```python
from build123d import *

# Parameters (mm, degrees)
SKETCH_1_R          = 10
EXTRUDE_1_DEPTH     = 3
SKETCH_2_R          = 1.5
CUT_EXTRUDE_1_DEPTH = 15.45683229480096
EXTRUDE_START       = 12.9
SKETCH_3_R          = 4.5
SKETCH_3_R_2        = 1.5000000000000002
EXTRUDE_2_DEPTH     = 12.9
EXTRUDE_START_2     = -15.9
SKETCH_4_R          = 1.5000000000000002
EXTRUDE_4_DEPTH     = 15.9
EXTRUDE_5_DEPTH     = 5
SKETCH_6_R          = 1.4999999999999751
CUT_EXTRUDE_2_DEPTH = 69.71105565006431
EXTRUDE_START_3     = 5
EXTRUDE_8_DEPTH     = 5
FILLET_1_R          = 10
FILLET_2_R          = 2
SKETCH_8_R          = 3.75
CUT_EXTRUDE_3_DEPTH = 3


with BuildPart() as part:
    # 草图1 → 凸台-拉伸1 (new body)
    with BuildSketch(Plane.XY):
        Circle(SKETCH_1_R)
    extrude(amount=EXTRUDE_1_DEPTH)

    # 草图2 → 切除-拉伸1 (cut, through all)
    with BuildSketch(Plane.XY.offset(3)):
        with BuildLine():
            ThreePointArc((-3.4499999999999966, 4.9499999999999975), (-6.010660171779826, 6.010660171779813), (-4.949999999999979, 3.4499999999999966))
            Line((-4.9499999999999975, 3.4499999999999966), (-4.9499999999999975, 4.949999999999997))
            Line((-4.9499999999999975, 4.9499999999999975), (-3.4499999999999957, 4.9499999999999975))
        make_face()
        with BuildLine():
            Line((-4.9499999999999975, 4.949999999999997), (-4.9499999999999975, 3.4499999999999966))
            ThreePointArc((-4.949999999999979, 3.4499999999999966), (-3.8893398282201694, 3.889339828220182), (-3.4499999999999966, 4.9499999999999975))
            Line((-3.4499999999999957, 4.9499999999999975), (-4.9499999999999975, 4.9499999999999975))
        make_face()
        with BuildLine():
            ThreePointArc((3.450000000000002, 4.95), (3.889339828220187, 3.889339828220172), (4.9500000000000215, 3.4499999999999993))
            Line((4.950000000000003, 3.4499999999999984), (4.950000000000003, 4.95))
            Line((4.950000000000003, 4.95), (3.450000000000002, 4.95))
        make_face()
        with BuildLine():
            Line((4.950000000000003, 4.95), (4.950000000000003, 3.4499999999999984))
            ThreePointArc((4.9500000000000215, 3.4499999999999993), (6.010660171779831, 3.8893398282201845), (6.450000000000004, 4.95))
            ThreePointArc((6.450000000000004, 4.95), (4.950000000000003, 6.450000000000001), (3.450000000000002, 4.95))
            Line((3.450000000000002, 4.95), (4.950000000000003, 4.95))
        make_face()
        with BuildLine():
            ThreePointArc((-4.949999999999978, -3.450000000000001), (-6.0106601717798265, -6.010660171779817), (-3.4499999999999966, -4.950000000000002))
            Line((-3.4499999999999957, -4.950000000000002), (-4.9499999999999975, -4.950000000000002))
            Line((-4.9499999999999975, -4.950000000000002), (-4.9499999999999975, -3.450000000000001))
        make_face()
        with BuildLine():
            Line((-4.9499999999999975, -4.950000000000002), (-3.4499999999999957, -4.950000000000002))
            ThreePointArc((-3.4499999999999966, -4.950000000000002), (-3.8893398282201685, -3.889339828220187), (-4.949999999999978, -3.450000000000001))
            Line((-4.9499999999999975, -3.450000000000001), (-4.9499999999999975, -4.950000000000002))
        make_face()
        with BuildLine():
            ThreePointArc((4.950000000000022, -3.4499999999999993), (3.889339828220188, -3.8893398282201717), (3.450000000000002, -4.95))
            Line((3.450000000000002, -4.95), (4.950000000000003, -4.95))
            Line((4.950000000000003, -4.95), (4.950000000000003, -3.4499999999999993))
        make_face()
        with BuildLine():
            Line((4.950000000000003, -4.95), (3.450000000000002, -4.95))
            ThreePointArc((3.450000000000002, -4.95), (4.950000000000003, -6.450000000000001), (6.450000000000004, -4.95))
            ThreePointArc((6.450000000000004, -4.95), (6.010660171779832, -3.8893398282201854), (4.950000000000022, -3.4499999999999993))
            Line((4.950000000000003, -3.4499999999999993), (4.950000000000003, -4.95))
        make_face()
        Circle(SKETCH_2_R)
    extrude(amount=-CUT_EXTRUDE_1_DEPTH, mode=Mode.SUBTRACT)

    # 草图3 → 凸台-拉伸2 (add)
    with BuildSketch(Plane.XY.offset(3).offset(EXTRUDE_START)):
        with Locations(Location((0, 0, 0), (0, 0, 180))):
            Circle(SKETCH_3_R)
        Circle(SKETCH_3_R_2, mode=Mode.SUBTRACT)
    extrude(amount=-EXTRUDE_2_DEPTH)

    # 草图4 → 凸台-拉伸4 (add)
    with BuildSketch(Plane(origin=(0, 0, 0), x_dir=(-1, 0, 0), z_dir=(0, 0, -1)).offset(EXTRUDE_START_2)):
        Circle(SKETCH_4_R)
    extrude(amount=EXTRUDE_4_DEPTH)

    # 草图5 → 凸台-拉伸5 (add)
    with BuildSketch(Plane.XY.offset(15.9)):
        Polygon((64.59529016246847, -5.1146065812479), (63.94313316774814, -10.575805282470675), (-0.5983060285210257, -2.8684953448666564), (0.05385096619931135, 2.5927033563560817), align=None)
    extrude(amount=EXTRUDE_5_DEPTH)

    # 草图6 → 切除-拉伸2 (cut, through all)
    with BuildSketch(Plane.XY.offset(20.900000000000002)):
        with Locations((59.55641321806875, -7.28242024320529)):
            Circle(SKETCH_6_R)
    extrude(amount=-CUT_EXTRUDE_2_DEPTH, mode=Mode.SUBTRACT)

    # 草图7 → 凸台-拉伸8 (add)
    with BuildSketch(Plane.XY.offset(15.9).offset(EXTRUDE_START_3)):
        with BuildLine():
            Line((0.05385096619931135, 2.5927033563560817), (3.9664004294167037, 2.1254805653129325))
            ThreePointArc((3.9664004294167037, 2.1254805653129325), (-4.4378387444626375, 0.7453772723569406), (3.054352769395848, -3.3046829136974565))
            Line((3.054352769395848, -3.3046829136974565), (-0.5983060285210257, -2.8684953448666564))
            Line((-0.5983060285210257, -2.8684953448666564), (0.05385096619931135, 2.5927033563560817))
        make_face()
    extrude(amount=-EXTRUDE_8_DEPTH)

    # 圆角1
    fillet_1_edges = [part.edges().sort_by_distance(p)[0] for p in [
        (4.437838744462656, -0.7453772723568349, 15.9),
    ]]
    fillet(fillet_1_edges, radius=FILLET_1_R)

    # 圆角2
    fillet_2_edges = [part.edges().sort_by_distance(p)[0] for p in [
        (63.94313316774814, -10.575805282470675, 18.4),
        (64.59529016246847, -5.1146065812479, 18.4),
    ]]
    fillet(fillet_2_edges, radius=FILLET_2_R)

    # 草图8 → 切除-拉伸3 (cut)
    with BuildSketch(Plane(origin=(0, 0, 0), x_dir=(-1, 0, 0), z_dir=(0, 0, -1))):
        Circle(SKETCH_8_R)
    extrude(amount=-CUT_EXTRUDE_3_DEPTH, mode=Mode.SUBTRACT)


solid = part.part
```
Here's how the part is built. I have some questions about the finished solid (model axes, mm). A direction names the side the tool comes from. Coordinates: 2 decimals unless noted, no trailing zeros. Order: outer loops, then holes, each group sorted by start corner. A loop starts at its lowest first (then second) coordinate and runs counter-clockwise, first axis right, second up.
Item 1: I need wall thicknesses on probe 1 along Y at (x, z) = (0, 1.55); probe 2 along Z at (x, y) = (29.5, -1.75); probe 3 along X at (y, z) = (-2, 14.25). Which ranges of each line are inside material? Lowest first, please.
Response values:
probe 1: y = -10 to -3.75, 3.75 to 10
probe 2: z = 15.9 to 20.9
probe 3: x = -4.03 to 8.77
Item 2: Thinking about a two-plate mould opening in X: for faces 1 (the face through (30.98, -1.1, 18.36)), 2 (the face through (4.3, -2.1, 3)), 3 (the face through (-4.144, -3.685, 1.521)), which applies, pulls with the +X half, pulls with the -X half, needs draft (parallel to the pull), parting line crosses it, or undercut?
Response values:
face 1: pulls with the +X half
face 2: needs draft
face 3: undercut
Item 3: Which directions (+Z, -Z, +X, -X, +Y, -Y) give clear straight access to the entire face, cutting with the end or side of a thin tool? Please do faces 4 (the face through (22, -3, 20.9)), 5 (the face through (39, -5, 15.9)), 6 (the face through (30.462, -6.578, 17.809)), 7 (the face through (3.746, 0.165, 1.479)).
Response values:
face 4: +Z, +X, -X, +Y, -Y
face 5: -Z, +X, +Y, -Y
face 6: +Z, -Y
face 7: -Z
Item 4: If we section it at D-D, the plane z = 14.75: List the corners of the cut face in (x, y) for me, then the cut area to 3 significant figures.
Response values:
outline: (3.05, -3.3) - (8.99, -4.01) arc R9.84 ccw to (9.74, 1.44) - (3.97, 2.13) arc R4.5 ccw (long way) to start
area: 94.0 mm2
Item 5: If we section it at B-B, the plane y = 0: List the corners of the cut face in (x, z) for me, then the cut area to 3 significant figures.
Response values:
outline: (-10, 0) - (-3.75, 0) - (-3.75, 3) - (3.75, 3) - (3.75, 0) - (10, 0) - (10, 3) - (4.5, 3) - (4.5, 5.9) arc R10 cw to (14.5, 15.9) - (21.77, 15.9) - (21.77, 20.9) - (-4.5, 20.9) - (-4.5, 3) - (-10, 3) - close
area: 306 mm2
Item 6: If we section it at C-C, the plane z = 4.5: List the corners of the cut face in (x, y) for me.
Response values:
outline: circle Ø9 at (0, 0)
Item 7: I'm going to push flat-ended pins straight in: pin 1 Ø12 at (x, z) = (39, 17) entering from +Y; pin 2 Ø5 at (y, z) = (3, 3.5) entering from -X; pin 3 Ø5 at (y, z) = (0.5, 8.5) entering from +X. Where does each tip first touch, or does it pass through?
Response values:
pin 1: stops at y = -1.34
pin 2: stops at x = -9.98
pin 3: stops at x = 5.89
Item 8: If we section it at A-A, the plane x = 0: List the corners of the cut face in (y, z) for me.
Response values:
outline: (-10, 0) - (-3.75, 0) - (-3.75, 3) - (3.75, 3) - (3.75, 0) - (10, 0) - (10, 3) - (4.5, 3) - (4.5, 20.9) - (-4.5, 20.9) - (-4.5, 3) - (-10, 3) - close
